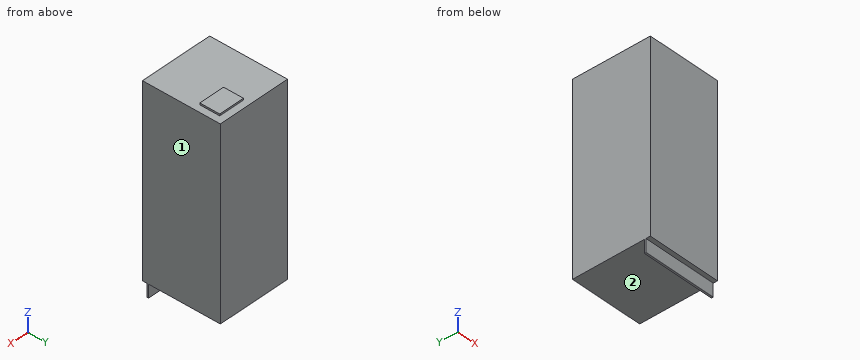
from build123d import *

# Parameters (mm, degrees)
SZKIC1_W                    = 85
SZKIC1_H                    = 90
DODANIE_WYCI_GNI_CIE1_DEPTH = 215
SZKIC2_W                    = 85
SZKIC2_H                    = 2
DODANIE_WYCI_GNI_CIE2_DEPTH = 15
SZKIC3_W                    = 30
SZKIC3_H                    = 23
DODANIE_WYCI_GNI_CIE3_DEPTH = 2


with BuildPart() as part:
    # Szkic1 → Dodanie-wyciągnięcie1 (new body)
    with BuildSketch(Plane.XY):
        Rectangle(SZKIC1_W, SZKIC1_H)
    extrude(amount=DODANIE_WYCI_GNI_CIE1_DEPTH)

    # Szkic2 → Dodanie-wyciągnięcie2 (add)
    with BuildSketch(Plane(origin=(0, 0, 0), x_dir=(-1, 0, 0), z_dir=(0, 0, -1))):
        with Locations((0, -39)):
            Rectangle(SZKIC2_W, SZKIC2_H)
    extrude(amount=DODANIE_WYCI_GNI_CIE2_DEPTH)

    # Szkic3 → Dodanie-wyciągnięcie3 (add)
    with BuildSketch(Plane.XY.offset(215)):
        with Locations((19.5, 25.5)):
            Rectangle(SZKIC3_W, SZKIC3_H)
    extrude(amount=DODANIE_WYCI_GNI_CIE3_DEPTH)


solid = part.part
For this review, take the finished solid that the model builds, in its own axes (mm). Face numbers are marked on the shaded views. A direction names the side the tool comes from. Round coordinates to 2 decimals unless told otherwise and drop trailing zeros. Loops run counter-clockwise (first coordinate to the right, second up) from the corner with the lowest first, then second, coordinate; pieces in that order, holes last. Notation, with made-up numbers: (-25, 18.25) - (14, 18.25) arc R30 ccw to (14, 50.25) - close; hole circle Ø1 at (60, 78). An arc over 180 degrees is marked (long way). Use one line per item in the form item = value.
Item 1: Consider section D-D on y = -15. Write out the cut boundary in (x, z).
Answers:
outline = (-42.5, 0) - (42.5, 0) - (42.5, 215) - (-42.5, 215) - close
Item 2: Consider section C-C on x = 20. Write out the cut boundary in (y, z).
Answers:
outline = (-45, 0) - (-40, 0) - (-40, -15) - (-38, -15) - (-38, 0) - (45, 0) - (45, 215) - (37, 215) - (37, 217) - (14, 217) - (14, 215) - (-45, 215) - close
Item 3: For line 1 (Z direction, x = -33, y = -28); line 2 (Y direction, x = -32, z = -3), list the stretches that pass through material, from the lowest coordinate up.
Answers:
line_1 = 0 to 215
line_2 = -40 to -38
Item 4: Tool access review of the marked faces 1 and 2: name each direction out of +Z, -Z, +X, -X, +Y, -Y from which nothing blocks a thin tool from reaching the whole face with its end or side.
Answers:
face_1 = +Z, -Z, +X, +Y, -Y
face_2 = -Z, +X, -X, +Y
Item 5: Consider section A-A on x = -24. Write out the cut boundary in (y, z), then the cut area to 3 significant figures.
Answers:
outline = (-45, 0) - (-40, 0) - (-40, -15) - (-38, -15) - (-38, 0) - (45, 0) - (45, 215) - (-45, 215) - close
area = 19,400 mm^2
Item 6: Clearance check with flat-ended pins moving along their axes: P1, Ø12, axis at x = -26.5, y = -14, coming from the -Z side; P2, Ø1, axis at y = 20, z = 216, coming from the -X side; P3, Ø0.6, axis at x = 21, z = 216, coming from the -Y side. State where each tip first meets the part, or that it passes through.
Answers:
P1 = 0
P2 = 4.5
P3 = 14
Item 7: Consider section B-B on y = 17.5. Write out the cut boundary in (x, z), then the cut area to 3 significant figures.
Answers:
outline = (-42.5, 0) - (42.5, 0) - (42.5, 215) - (34.5, 215) - (34.5, 217) - (4.5, 217) - (4.5, 215) - (-42.5, 215) - close
area = 18,300 mm^2
